Geometry: see drawing. Coordinates: mm, zero at the bounding-box minimum. A direction names the side the tool comes from. Coordinates: 2 decimals unless noted, no trailing zeros. Order: outer loops, then holes, each group sorted by start corner. A loop starts at its lowest first (then second) coordinate and runs counter-clockwise, first axis right, second up. Notation, with made-up numbers: M 71.5,9 L 94.5,9 A12 cw 94.5,22 Z; hole C -24.5,60.25 d10. An arc over 180 degrees is marked long. One line per item, written item: value.
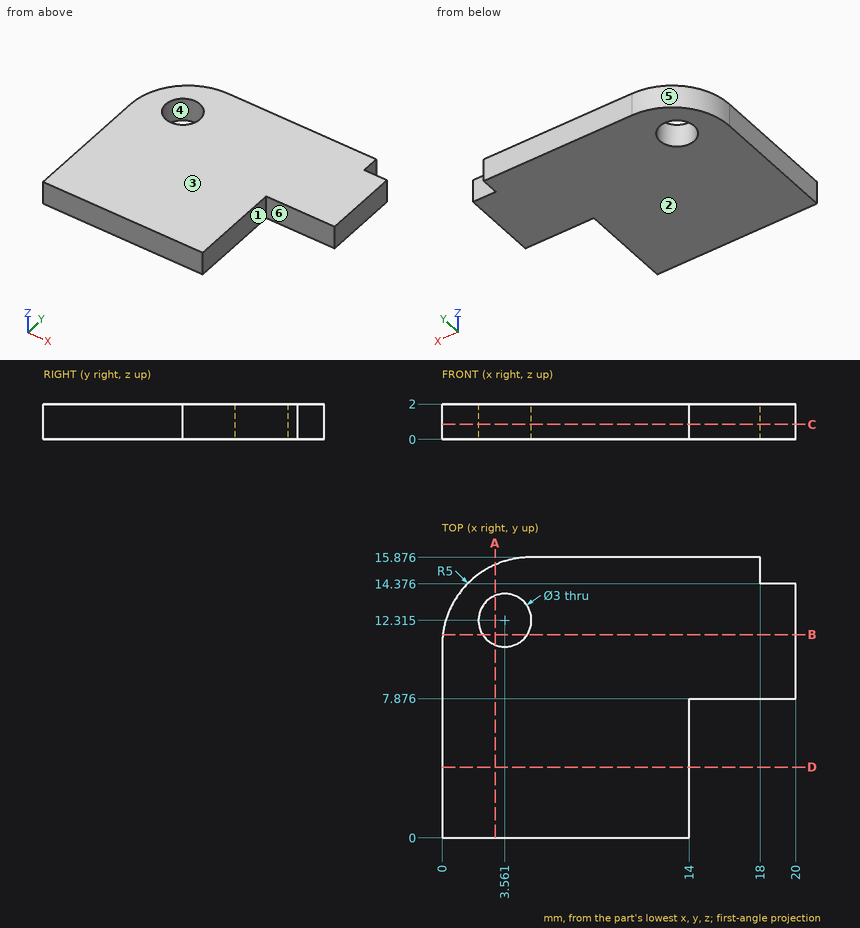
(1) Access query for the marked faces 1 and 2. Directions: +Z, -Z, +X, -X, +Y, -Y. A direction counts if a zero-diameter tool reaches every point of the face in a straight line with its end or side. Return the directions, or none.
Data:
face 1: +Z, -Z, +X, -Y
face 2: -Z, +X, -X, +Y, -Y
(2) First-contact query: pin 1 (1 mm diameter, centred on x = 17.5, z = 1.5, fed in from -Y). Flat tip, straight axial feed; report the tip coordinate or a pass-through.
Data:
pin 1: stops at y = 7.88
(3) Cut plane A-A on x = 3. Output: boundary loops of the cut face in (y, z).
Data:
outline: M 0,0 L 10.92,0 L 10.92,2 L 0,2 Z; M 13.71,0 L 15.46,0 L 15.46,2 L 13.71,2 Z
(4) Cut plane C-C on z = 0.85. Output: boundary loops of the cut face in (x, y) (1 decimal).
Data:
outline: M 0,0 L 14,0 L 14,7.9 L 20,7.9 L 20,14.4 L 18,14.4 L 18,15.9 L 5,15.9 A5 ccw 0,10.9 Z; hole C 3.6,12.3 d3
(5) Cut plane B-B on y = 11.5. Output: boundary loops of the cut face in (x, z).
Data:
outline: M 0.04,0 L 2.3,0 L 2.3,2 L 0.04,2 Z; M 4.82,0 L 20,0 L 20,2 L 4.82,2 Z
(6) Ray query, line 1 (X direction, y = 2.5, z = 0.45); line 2 (X direction, y = 13.5, z = 0.75) (1 decimal); line 3 (Y direction, x = 16.5, z = 1.1) (1 decimal). Return the intervals inside material, ascending. Write a range as from..to.
Data:
line 1: x = 0..14
line 2: x = 0.7..2.6, 4.5..20
line 3: y = 7.9..15.9
(7) Cut plane D-D on y = 4. Output: boundary loops of the cut face in (x, z), plus the area to 3 significant figures.
Data:
outline: M 0,0 L 14,0 L 14,2 L 0,2 Z
area: 28.0 mm2
(8) Draft query along Y for the marked faces 3, 4, 5 and 6. Return one class per face: released by +Y, released by -Y, zero draft, split by the parting line, or undercut.
Data:
face 3: zero draft
face 4: undercut
face 5: released by +Y
face 6: released by -Y
